Geometry check sheet. Reference: the model listing, model coordinates, mm. Give positions to 0.01 mm unless a question says otherwise; leave off trailing zeros. Write each loop counter-clockwise with the first axis right and the second up, starting at its lowest first coordinate (ties: lowest second). Pieces come first, ordered by that corner, then holes. Notation, with made-up numbers: M -14,-17.5 L -9,-17.5 A24 ccw -9,-0.5 Z; hole C 57.5,79 d5. An arc over 180 degrees is marked long. One line per item, written item: value. Start each with the question number.
1. Cross-section at A-A on y = 0. Record the cut outline in (x, z) (3 decimals).
2. Scan lines: line 1 (Y direction, x = -73.25, z = 0); line 2 (Y direction, x = -73.75, z = 4); line 3 (Z direction, x = -73.3, y = 1.5). Record each from-to range of solid material in increasing order.
3. Cross-section at B-B on z = -5. Record the cut outline in (x, y) (3 decimals), then the cut area to 3 significant figures.
4. Cross-section at C-C on x = -72.35. Record the cut outline in (y, z).
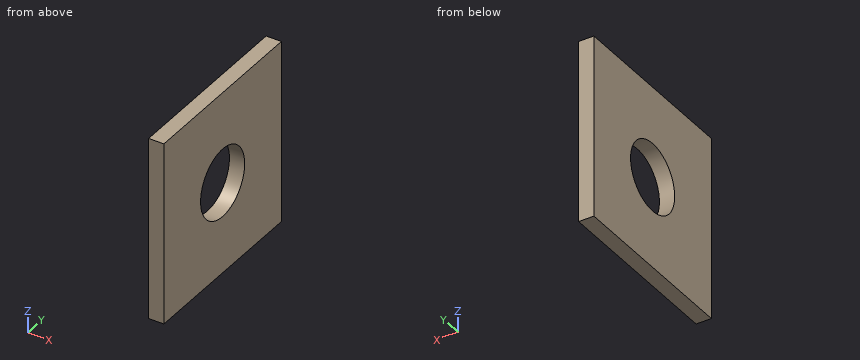
from build123d import *

# Parameters (mm, degrees)
SKETCH3_W                   = 3.175
SKETCH3_H                   = 38.1
APERTURE_PLATE_F_DEPTH      = 19.05
APERTURE_PLATE_F_DEPTH_BACK = 19.05
APERTURE_F_REACH            = 5.175
SKETCH6_R                   = 7.1501


with BuildPart() as part:
    # Sketch3 → APERTURE_PLATE_F (new body, two sides)
    with BuildSketch(Plane(origin=(0, 0, 0), x_dir=(1, 0, 0), z_dir=(0, 1, 0))) as aperture_plate_f_sk:
        with Locations((-72.7075, 0)):
            Rectangle(SKETCH3_W, SKETCH3_H)
    extrude(amount=APERTURE_PLATE_F_DEPTH)
    extrude(aperture_plate_f_sk.sketch, amount=-APERTURE_PLATE_F_DEPTH_BACK)

    # Sketch6 → APERTURE_F (cut, up to next)
    with BuildSketch(Plane(origin=(-71.12, 0, 0), x_dir=(0, 0, -1), z_dir=(1, 0, 0)), mode=Mode.PRIVATE) as aperture_f_sk1:
        Circle(SKETCH6_R)
    aperture_f_tool1 = extrude(aperture_f_sk1.sketch, amount=-APERTURE_F_REACH, mode=Mode.PRIVATE) & part.part
    add(aperture_f_tool1.solids().sort_by_distance((-71.12, 0, 0))[0], mode=Mode.SUBTRACT)


solid = part.part
Report:
1. outline: M -74.295,-19.05 L -71.12,-19.05 L -71.12,-7.15 L -74.295,-7.15 Z; M -74.295,7.15 L -71.12,7.15 L -71.12,19.05 L -74.295,19.05 Z
2. line 1: y = -19.05 to -7.15, 7.15 to 19.05
2. line 2: y = -19.05 to -5.93, 5.93 to 19.05
2. line 3: z = -19.05 to -6.99, 6.99 to 19.05
3. outline: M -74.295,-19.05 L -71.12,-19.05 L -71.12,-5.111 L -74.295,-5.111 Z; M -74.295,5.111 L -71.12,5.111 L -71.12,19.05 L -74.295,19.05 Z
3. area: 88.5 mm^2
4. outline: M -19.05,-19.05 L 19.05,-19.05 L 19.05,19.05 L -19.05,19.05 Z; hole C 0,0 d14.3
